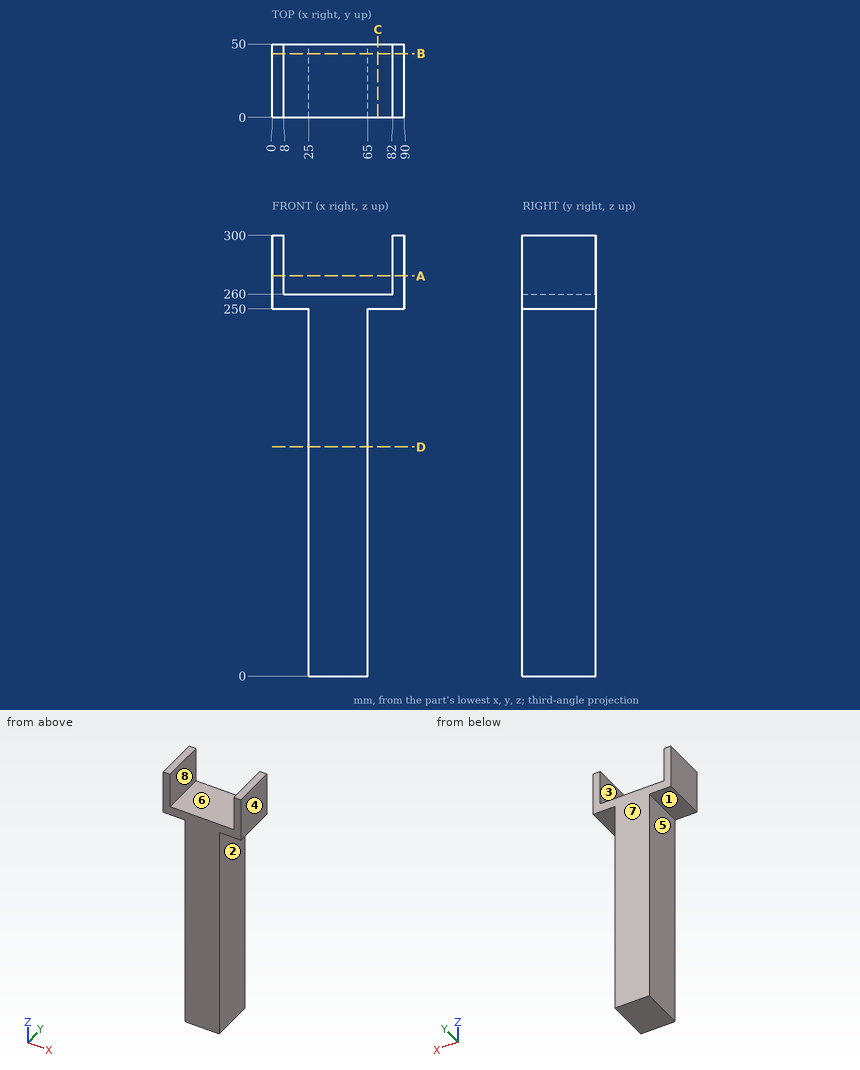
Drawing for the job (mm, zero at the part's lowest x, y, z). A direction names the side the tool comes from. Round coordinates to 2 decimals unless told otherwise and drop trailing zeros. Write each loop counter-clockwise with the first axis right and the second up, starting at its lowest first coordinate (ties: lowest second). Pieces come first, ordered by that corner, then holes. Notation, with made-up numbers: M 50,-9 L 105,-9 A16 ccw 105,5 Z; hole C 42.25,-0.75 d10. An arc over 180 degrees is marked long. Put each result on its own line as item: value.
Item 1: Mould opens along X. For the marked faces 5, 6, 7 and 8 say: +X half, -X half, draft (parallel to the pull), parting line (faces both ways), or undercut.
Responses:
face 5: -X half
face 6: undercut
face 7: draft
face 8: undercut
Item 2: Cut at C-C (x = 72). List the corners of the cut face in (y, z).
Responses:
outline: M 0,250 L 50,250 L 50,260 L 0,260 Z
Item 3: Flat gauge pins, fed straight in: P1, Ø12, axis at y = 42, z = 86.5, coming from the -X side; P2, Ø12, axis at y = 25, z = 164, coming from the +X side; P3, Ø7.5, axis at x = 10, y = 13.5, coming from the -Z side. Where does each tip first touch, or does it go through?
Responses:
P1: x = 25
P2: x = 65
P3: z = 250
Item 4: Cut at B-B (y = 43.5). List the corners of the cut face in (x, z).
Responses:
outline: M 0,250 L 25,250 L 25,0 L 65,0 L 65,250 L 90,250 L 90,300 L 82,300 L 82,260 L 8,260 L 8,300 L 0,300 Z
Item 5: Probe L1, parallel to X at y = 9.5, z = 183.5; L2, parallel to Z at x = 54, y = 3; L3, parallel to Z at x = 14, y = 20. List the from-to ranges inside material, lowest first. Write a range as from..to.
Responses:
L1: 25..65
L2: 0..260
L3: 250..260
Item 6: Cut at A-A (z = 272.5). List the corners of the cut face in (x, y).
Responses:
outline: M 0,0 L 8,0 L 8,50 L 0,50 Z; M 82,0 L 90,0 L 90,50 L 82,50 Z
Item 7: Tool access for the marked faces 1, 2, 3 and 4: list every direction of +Z, -Z, +X, -X, +Y, -Y with a clear straight run to the whole face (end or side of a thin tool).
Responses:
face 1: -Z, -X, +Y, -Y
face 2: -Z, +X, +Y, -Y
face 3: +Z, +Y, -Y
face 4: +Z, -Z, +X, +Y, -Y
Item 8: Cut at D-D (z = 156). List the corners of the cut face in (x, y).
Responses:
outline: M 25,0 L 65,0 L 65,50 L 25,50 Z
